Answer from the drawing. Dimensions are ordinates in mm from the lowest x, y and z of the part. A direction names the side the tool comes from. Coordinates: 2 decimals unless noted, no trailing zeros. Order: outer loops, then holes, each group sorted by start corner. A loop starts at its lowest first (then second) coordinate and runs counter-clockwise, first axis right, second up. Notation, with made-up numbers: (18, -25) - (38, -25) arc R28 ccw to (38, 1) - close; hole circle Ø8 at (-1, 5). An arc over 180 degrees is marked (long way). Answer as a JSON object with one key per item and string values. Group by question number.
1) A tool of negligible diameter and unlimited length cuts with its end or side. For the marked faces 1, 2 and 3, from which of +Z, -Z, +X, -X, +Y, -Y can it reach the whole face along a straight path? Write none if from no direction.
2) Section D-D (z = 8.75) is taken. Give the vertices of the cut face in (x, y).
3) Section B-B (y = 12) is taken. Give the vertices of the cut face in (x, z).
4) Section C-C (x = 7.5) is taken. Give the vertices of the cut face in (y, z).
5) Find the intervals of material crossed by line 1 along Y through (x, z) = (12.6, 12.5); line 2 along Y through (x, z) = (22, 11); line 3 along X through (y, z) = (5, 12), in increasing order.
6) Each of these flat-tipped pins is pushed along its axis until it touches: P1, Ø1.2, axis at x = 17, z = 14, coming from the +Y side; P2, Ø1.5, axis at y = 7, z = 9, coming from the +X side; P3, Ø2, axis at y = 12, z = 12.5, coming from the -X side. Where does it stop, or does it pass through?
7) Section A-A (z = 2) is taken. Give the vertices of the cut face in (x, y).
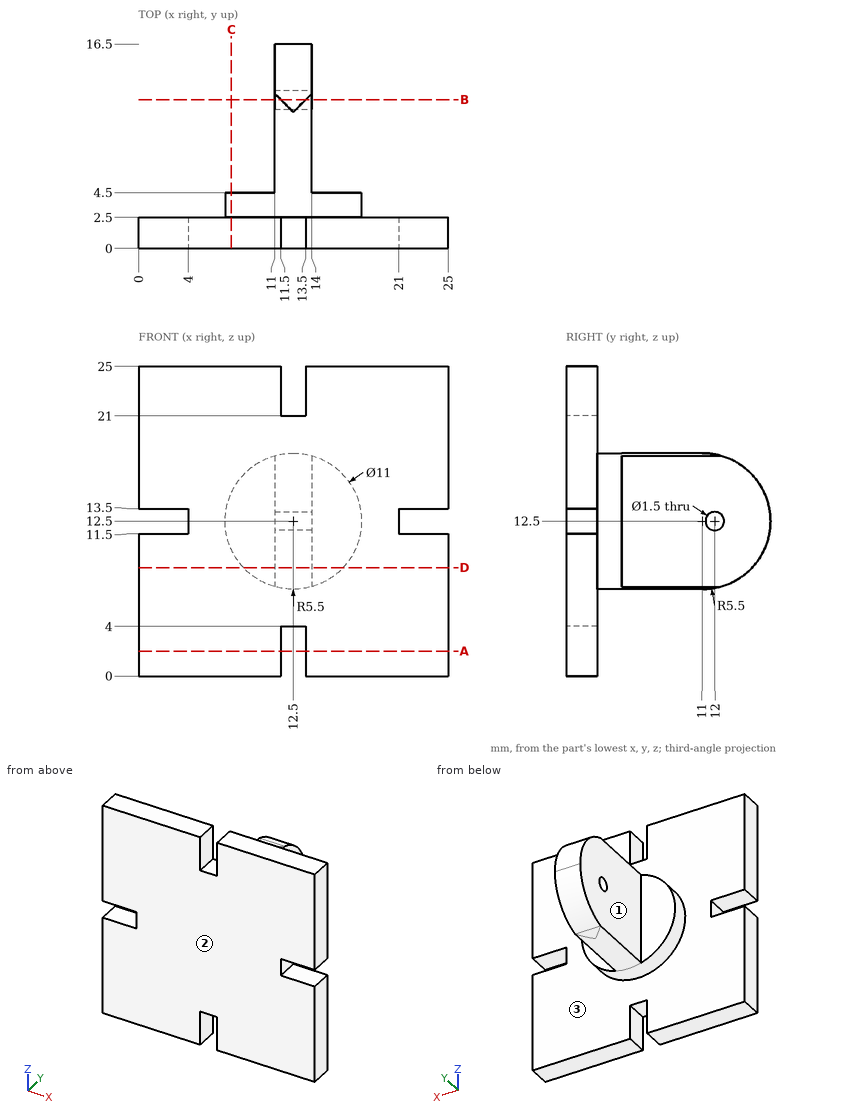
Report:
{
 "1": {"face 1": "+Z, -Z, -X, +Y", "face 2": "+Z, -Z, +X, -X, -Y", "face 3": "+Y"},
 "2": {"outline": "(0, 0) - (25, 0) - (25, 2.5) - (16.52, 2.5) - (16.52, 4.5) - (14, 4.5) - (14, 15.02) - (11, 15.02) - (11, 4.5) - (8.48, 4.5) - (8.48, 2.5) - (0, 2.5) - close"},
 "3": {"outline": "(11, 7.21) arc R5.5 ccw to (11.5, 7.09) - (13.5, 7.09) arc R5.5 ccw to (14, 7.21) - (14, 11.75) - (11, 11.75) - close; (11, 13.25) - (14, 13.25) - (14, 17.79) arc R5.5 ccw to (13.5, 17.91) - (11.5, 17.91) arc R5.5 ccw to (11, 17.79) - close"},
 "4": {"outline": "(0, 0) - (2.5, 0) - (2.5, 10.21) - (4.5, 10.21) - (4.5, 14.79) - (2.5, 14.79) - (2.5, 25) - (0, 25) - close"},
 "5": {"line 1": "y = 0 to 11.25, 12.75 to 16.5", "line 2": "y = 0 to 2.5", "line 3": "x = 11 to 14"},
 "6": {"P1": "stops at y = 4.5", "P2": "stops at x = 14", "P3": "stops at x = 11"},
 "7": {"outline": "(0, 0) - (11.5, 0) - (11.5, 2.5) - (0, 2.5) - close; (13.5, 0) - (25, 0) - (25, 2.5) - (13.5, 2.5) - close"}
}
